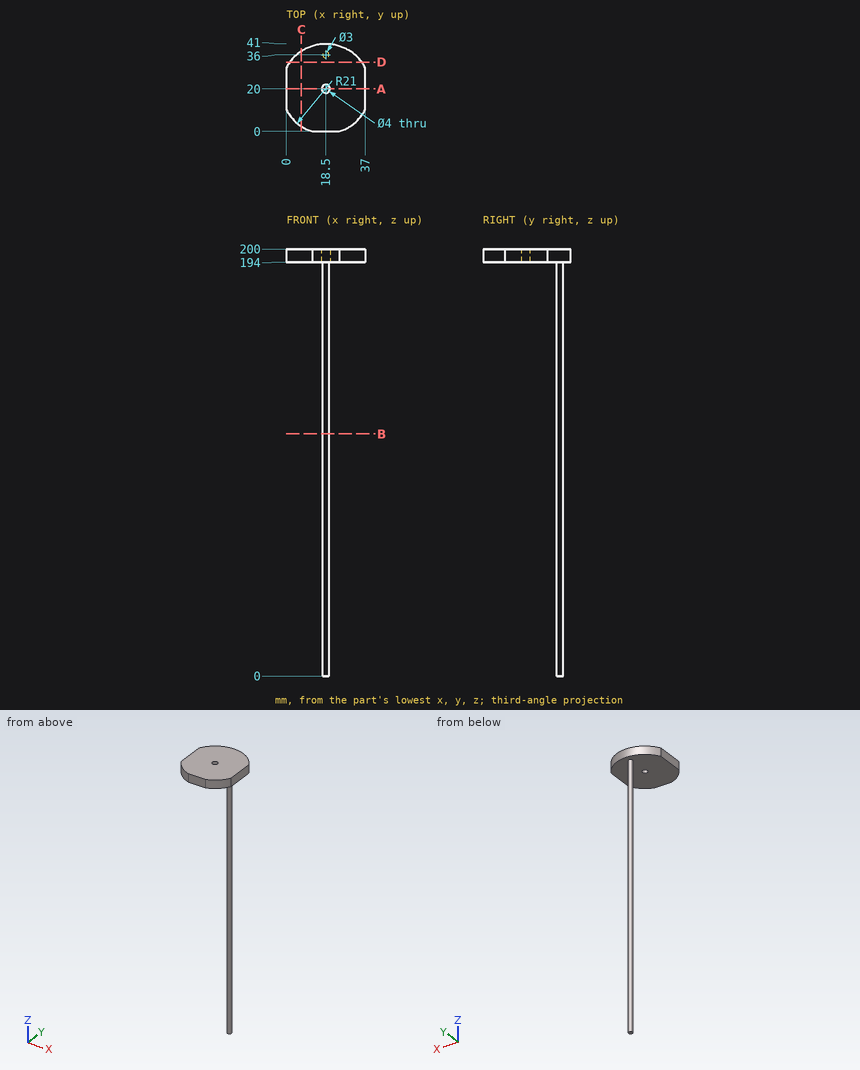
Part print with two shaded views. Sizes in mm from the minimum x, y, z corner. Give positions to 0.01 mm unless a question says otherwise; leave off trailing zeros. Order: outer loops, then holes, each group sorted by start corner. A loop starts at its lowest first (then second) coordinate and runs counter-clockwise, first axis right, second up. Notation, with made-up numbers: M -22,54.5 L -5,54.5 A23 cw -5,88.5 Z; hole C -6.75,79 d7. An arc over 180 degrees is marked long. Put each result on its own line as item: value.
Item 1: Cut at C-C on x = 7. Write the cut outline in (y, z).
Results are:
outline: M 2.43,194 L 37.57,194 L 37.57,200 L 2.43,200 Z
Item 2: Cut at A-A on y = 20. Write the cut outline in (x, z).
Results are:
outline: M 0,194 L 16.5,194 L 16.5,200 L 0,200 Z; M 20.5,194 L 37,194 L 37,200 L 20.5,200 Z
Item 3: Wall check: probe 1 along Y at (x, z) = (18, 196); probe 2 along Z at (x, y) = (11, 30.5); probe 3 along X at (y, z) = (35, 48.5). Give the ranges that are in metal, low to high.
Results are:
probe 1: 0 to 18.06, 21.94 to 40.99
probe 2: 194 to 200
probe 3: 17.38 to 19.62
Item 4: Cut at B-B on z = 113.5. Write the cut outline in (x, y).
Results are:
outline: C 18.5,36 d3
Item 5: Cut at D-D on y = 32.5. Write the cut outline in (x, z), then the cut area to 3 significant figures.
Results are:
outline: M 1.63,194 L 35.37,194 L 35.37,200 L 1.63,200 Z
area: 202 mm2
Item 6: Drop a flat-ended pin along its axis: pin 1 Ø1 at (x, y) = (12, 21) entering from -Z. Give the stop position or say it passes through.
Results are:
pin 1: z = 194
